Geometry: final body of the model. Coordinates: model frame, mm. Face numbers are marked on the shaded views. A direction names the side the tool comes from. Coordinates: 2 decimals unless noted, no trailing zeros. Write each loop counter-clockwise with the first axis right and the second up, starting at its lowest first coordinate (ties: lowest second). Pieces come first, ordered by that corner, then holes. Notation, with made-up numbers: (49, 53) -> (81, 53) arc R17 ccw to (81, 60) -> close; hole circle Ø9 at (12, 61). An arc over 180 degrees is marked (long way). One line per item, written item: value.
```python
from build123d import *

# Parameters (mm, degrees)
SKETCH_1_R          = 10
SKETCH_1_R_2        = 4.1
EXTRUDE_1_DEPTH     = 10
CUT_EXTRUDE_1_DEPTH = 18.320508076
SKETCH_3_R          = 1
CUT_EXTRUDE_2_DEPTH = 7
SKETCH_4_R          = 1.55
CUT_EXTRUDE_3_DEPTH = 11
SKETCH_5_W          = 5.5
SKETCH_5_H          = 2.5
CUT_EXTRUDE_4_DEPTH = 8


with BuildPart() as part:
    # 草图1 → 凸台-拉伸1 (new body)
    with BuildSketch(Plane(origin=(0, 0, 0), x_dir=(1, 0, 0), z_dir=(0, 1, 0))):
        with Locations(Location((0, 0, 0), (0, 0, 270))):
            Circle(SKETCH_1_R)
        with Locations(Location((0, 0, 0), (0, 0, 270))):
            Circle(SKETCH_1_R_2, mode=Mode.SUBTRACT)
    extrude(amount=EXTRUDE_1_DEPTH)

    # 草图2 → 切除-拉伸1 (cut, through all)
    with BuildSketch(Plane(origin=(0, 10, 0), x_dir=(1, 0, 0), z_dir=(0, 1, 0))):
        with BuildLine():
            Line((-6.5, -7.599342077), (6.5, -7.599342077))
            ThreePointArc((6.5, -7.599342077), (0, -10), (-6.5, -7.599342077))
        make_face()
    extrude(amount=-CUT_EXTRUDE_1_DEPTH, mode=Mode.SUBTRACT)

    # 草图3 → 切除-拉伸2 (cut)
    with BuildSketch(Plane.XY.offset(7.599342077)):
        with Locations((-3.5, 4.5)):
            Circle(SKETCH_3_R)
        with Locations((3, 4.5)):
            Circle(SKETCH_3_R)
    extrude(amount=-CUT_EXTRUDE_2_DEPTH, mode=Mode.SUBTRACT)

    # 草图4 → 切除-拉伸3 (cut)
    with BuildSketch(Plane.XY.offset(-2.400657923)):
        with Locations((0, 5.148756005)):
            Circle(SKETCH_4_R)
    extrude(amount=-CUT_EXTRUDE_3_DEPTH, mode=Mode.SUBTRACT)

    # 草图5 → 切除-拉伸4 (cut)
    with BuildSketch(Plane(origin=(0, 10, 0), x_dir=(1, 0, 0), z_dir=(0, 1, 0))):
        with Locations((-0.049141686, 6.782816016)):
            Rectangle(SKETCH_5_W, SKETCH_5_H)
    extrude(amount=-CUT_EXTRUDE_4_DEPTH, mode=Mode.SUBTRACT)


solid = part.part
```
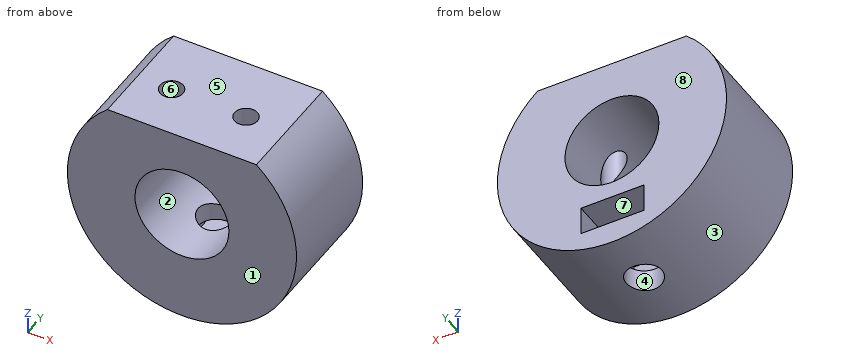
(1) Pull-direction query (X, two-part tool) for the marked faces 1, 2 and 3; classes: released by +X, released by -X, zero draft, split by the parting line, or undercut.
Responses:
face 1: zero draft
face 2: undercut
face 3: split by the parting line
(2) Section B-B (z = 0). Return the cut outline in (x, y), then the cut area to 3 significant figures.
Responses:
outline: (-10, 0) -> (-4.1, 0) -> (-4.1, 10) -> (-10, 10) -> close; (4.1, 0) -> (10, 0) -> (10, 10) -> (4.1, 10) -> close
area: 118 mm2
(3) Reachability of the marked faces 4, 5, 6, 7 and 8 from +Z, -Z, +X, -X, +Y, -Y: full face, straight path, thin tool, end or side. Return the list, or none.
Responses:
face 4: -Z
face 5: +Z, +X, -X, +Y, -Y
face 6: +Z
face 7: +Y
face 8: +Z, -Z, +X, -X, +Y
(4) Section D-D (x = 3). Return the cut outline in (y, z), then the cut area to 3 significant figures.
Responses:
outline: (0, -9.54) -> (10, -9.54) -> (10, -2.79) -> (0, -2.79) -> close; (0, 2.79) -> (3.5, 2.79) -> (3.5, 7.6) -> (0, 7.6) -> close; (5.5, 2.79) -> (10, 2.79) -> (10, 7.6) -> (5.5, 7.6) -> close
area: 106 mm2
(5) First-contact query: pin 1 (4 mm diameter, centred on y = 8.5, z = -6.5, fed in from -X); pin 2 (6 mm diameter, centred on x = -4.5, y = 5, fed in from -Z); pin 3 (2 mm diameter, centred on y = 4.5, z = -6.5, fed in from -X); pin 4 (6.5 mm diameter, centred on x = 0, z = 0, fed in from +Y). Flat tips, straight axial feed; report the tip coordinate or a pass-through.
Responses:
pin 1: stops at x = -8.93
pin 2: stops at z = -9.89
pin 3: stops at x = -8.35
pin 4: passes through
(6) Section C-C (y = 9.25). Return the cut outline in (x, z).
Responses:
outline: (-6.5, 7.6) arc R10 ccw (long way) to (6.5, 7.6) -> close; hole circle Ø8.2 at (0, 0); hole (-2.8, -8.03) -> (2.7, -8.03) -> (2.7, -5.53) -> (-2.8, -5.53) -> close
(7) Line query: line 1 (Z direction, x = 0, y = 7.75); line 2 (Y direction, x = 3, z = 3.75); line 3 (Y direction, x = 0, z = -4.6). Output: solid intervals per line, ascending. Write a range as [from, to].
Responses:
line 1: z = [-10, -8.03], [-5.53, -4.1], [4.1, 7.6]
line 2: y = [0, 3.5], [5.5, 10]
line 3: y = [0, 3.6], [6.7, 10]
(8) Section A-A (x = 0). Return the cut outline in (y, z), then the cut area to 3 significant figures.
Responses:
outline: (0, -10) -> (3.6, -10) -> (3.6, -8.03) -> (2, -8.03) -> (2, -5.53) -> (3.6, -5.53) -> (3.6, -4.1) -> (0, -4.1) -> close; (0, 4.1) -> (10, 4.1) -> (10, 7.6) -> (0, 7.6) -> close; (6.7, -10) -> (10, -10) -> (10, -8.03) -> (6.7, -8.03) -> close; (6.7, -5.53) -> (10, -5.53) -> (10, -4.1) -> (6.7, -4.1) -> close
area: 63.5 mm2
